Part model, mm, in its own coordinate system. Give positions to 0.01 mm unless a question says otherwise; leave off trailing zeros. Order: outer loops, then holes, each group sorted by start corner. A loop starts at its lowest first (then second) coordinate and runs counter-clockwise, first axis right, second up.
1. Slice it at C-C on x = 3.5. List the corners of the cut face in (y, z), and give its area (3 significant figures).
2. Slice it at B-B on z = 3.25. List the corners of the cut face in (x, y), and give its area (3 significant figures).
3. Slice it at D-D on x = 12.5. List the corners of the cut face in (y, z), and give its area (3 significant figures).
4. Slice it at A-A on x = 0. List the corners of the cut face in (y, z).
5. Probe line 1 (Y direction, x = -0.5, z = 6.5); line 2 (Y direction, x = 5, z = 0.5); line 3 (X direction, y = -0.5, z = 3). List the from-to ranges inside material, lowest first.
6. Drop flat-ended pins along their axis: pin 1 Ø3 at (x, z) = (-7.5, 4) entering from -Y; pin 2 Ø5 at (x, z) = (3.5, 7) entering from +Y; pin 3 Ø6 at (x, z) = (-6.5, 5.5) entering from -Y. Give the stop position or say it passes through.
from build123d import *
from build123d.topology import SkipClean

# Parameters (mm, degrees)
BOSS_EXTRUDE1_DEPTH = 10


with BuildPart() as part:
    # Sketch1 → Boss-Extrude1 (new body)
    # profile 1 of 2: a face of its own
    with SkipClean():  # the faces are left unmerged after this step: merging them gives an invalid solid
        with BuildSketch(Plane.XY):
            with BuildLine():
                Line((-15, 0), (-15, -50))
                ThreePointArc((-15, -50), (0, -65), (15, -50))
                Line((15, -50), (15, 0))
                ThreePointArc((15, 0), (0, 15), (-15, 0))
            make_face()
            with BuildLine():
                ThreePointArc((-10.25, -50), (0, -60.25), (10.25, -50))
                Line((10.25, -50), (10.25, 0))
                ThreePointArc((10.25, 0), (0, 10.25), (-10.25, 0))
                Line((-10.25, 0), (-10.25, -50))
            make_face(mode=Mode.SUBTRACT)
        # profile 2 of 2: a face of its own
        with BuildSketch(Plane.XY):
            with BuildLine():
                Line((10.25, -50), (10.25, 0))
                ThreePointArc((10.25, 0), (0, -10.25), (-10.25, 0))
                Line((-10.25, 0), (-10.25, -50))
                ThreePointArc((-10.25, -50), (0, -39.75), (10.25, -50))
            make_face()
        extrude(amount=BOSS_EXTRUDE1_DEPTH)
    add(part.part.scale(1), mode=Mode.REPLACE)  # the faces are merged on a copy


solid = part.part
Data:
1. outline: (-64.59, 0) - (-59.63, 0) - (-59.63, 10) - (-64.59, 10) - close; (-40.37, 0) - (-9.63, 0) - (-9.63, 10) - (-40.37, 10) - close; (9.63, 0) - (14.59, 0) - (14.59, 10) - (9.63, 10) - close
1. area: 406 mm2
2. outline: (-15, -50) arc R15 ccw to (15, -50) - (15, 0) arc R15 ccw to (-15, 0) - close; hole circle Ø20.5 at (0, -50); hole circle Ø20.5 at (0, 0)
2. area: 1,550 mm2
3. outline: (-58.29, 0) - (8.29, 0) - (8.29, 10) - (-58.29, 10) - close
3. area: 666 mm2
4. outline: (-65, 0) - (-60.25, 0) - (-60.25, 10) - (-65, 10) - close; (-39.75, 0) - (-10.25, 0) - (-10.25, 10) - (-39.75, 10) - close; (10.25, 0) - (15, 0) - (15, 10) - (10.25, 10) - close
5. line 1: y = -64.99 to -60.24, -39.76 to -10.24, 10.24 to 14.99
5. line 2: y = -64.14 to -58.95, -41.05 to -8.95, 8.95 to 14.14
5. line 3: x = -15 to -10.24, 10.24 to 15
6. pin 1: stops at y = -63.75
6. pin 2: stops at y = 14.97
6. pin 3: stops at y = -64.59
